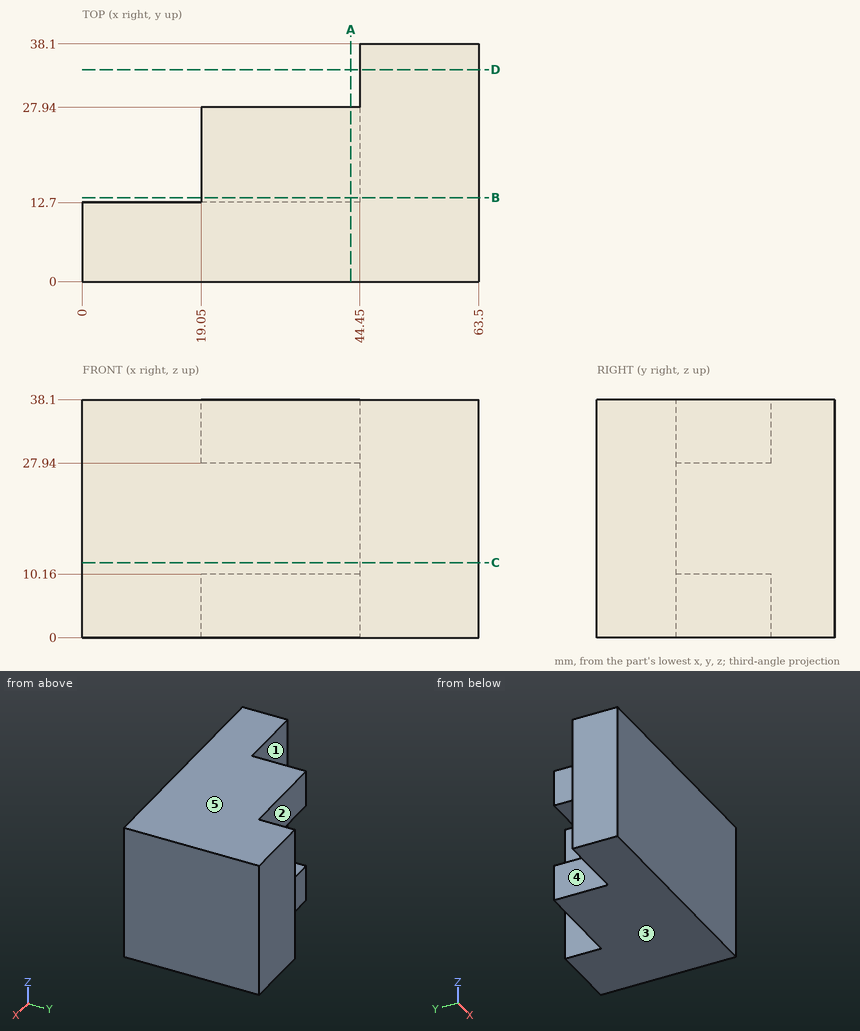
Verification items for this drawing (mm, ordinates from the low corner). A direction names the side the tool comes from. Give positions to 0.01 mm unless a question says otherwise; leave off trailing zeros. Loops run counter-clockwise (first coordinate to the right, second up) from the corner with the lowest first, then second, coordinate; pieces in that order, holes last. Notation, with made-up numbers: M 10,-3 L 53,-3 A31 cw 53,25 Z; hole C 11.25,-5.75 d9. An arc over 180 degrees is marked long. Write item = value, one per line. Start each with the question number.
1. Section check C-C, the plane z = 12. Enter the section's corners in (x, y).
2. Section check D-D, the plane y = 34. Enter the section's corners in (x, z), plus the area to 3 significant figures.
3. Thickness scan on probe 1 along Z at (x, y) = (38, 23); probe 2 along Y at (x, z) = (4, 14.5); probe 3 along X at (y, z) = (23.5, 22). Record the ranges inside material, lowest first.
4. Tool access check on the marked faces 4 and 5. Record the directions out of +Z, -Z, +X, -X, +Y, -Y that give a thin tool (end or side, any length) a straight path to the whole face; none if there is none.
5. Go/stop test with flat-tipped pins: P1, Ø4, axis at x = 39.5, z = 21.5, coming from the +Y side; P2, Ø5, axis at x = 36, z = 4.5, coming from the +Y side; P3, Ø12, axis at x = 11.5, y = 21, coming from the +Z side; P4, Ø3, axis at y = 18.5, z = 32, coming from the -X side. Record where each tip stops, or that it passes through.
6. Section check A-A, the plane x = 43. Enter the section's corners in (y, z).
7. Section check B-B, the plane y = 13.5. Enter the section's corners in (x, z).
8. Draft check along Z on the marked faces 1, 2 and 3. Enter one of: +Z half, -Z half, draft (parallel to the pull), parting line (faces both ways), or undercut.
Values follow:
q1.outline = M 0,0 L 63.5,0 L 63.5,38.1 L 44.45,38.1 L 44.45,12.7 L 0,12.7 Z
q2.outline = M 44.45,0 L 63.5,0 L 63.5,38.1 L 44.45,38.1 Z
q2.area = 726 mm^2
q3.probe_1 = 0 to 10.16, 27.94 to 38.1
q3.probe_2 = 0 to 12.7
q3.probe_3 = 44.45 to 63.5
q4.face_4 = +Z, -Z, -X, +Y
q4.face_5 = +Z, +X, -X, +Y, -Y
q5.P1 = 12.7
q5.P2 = 27.94
q5.P3 = through
q5.P4 = 19.05
q6.outline = M 0,0 L 27.94,0 L 27.94,10.16 L 12.7,10.16 L 12.7,27.94 L 27.94,27.94 L 27.94,38.1 L 0,38.1 Z
q7.outline = M 19.05,0 L 63.5,0 L 63.5,38.1 L 19.05,38.1 L 19.05,27.94 L 44.45,27.94 L 44.45,10.16 L 19.05,10.16 Z
q8.face_1 = undercut
q8.face_2 = draft
q8.face_3 = -Z half
